Source: three-view drawing plus pictorial views. Frame: mm from the lowest corner of the part. A direction names the side the tool comes from. Give positions to 0.01 mm unless a question says otherwise; leave off trailing zeros. Write each loop counter-clockwise with the first axis right and the second up, starting at its lowest first coordinate (ties: lowest second). Pieces come first, ordered by that corner, then holes. Notation, with made-up numbers: (48.5, -31) - (76.5, -31) arc R13 ccw to (76.5, -10) - close; hole circle Ø9 at (85.5, 2). An arc over 180 degrees is marked (long way). One line per question, with ' | ' between items. Start each with the question number.
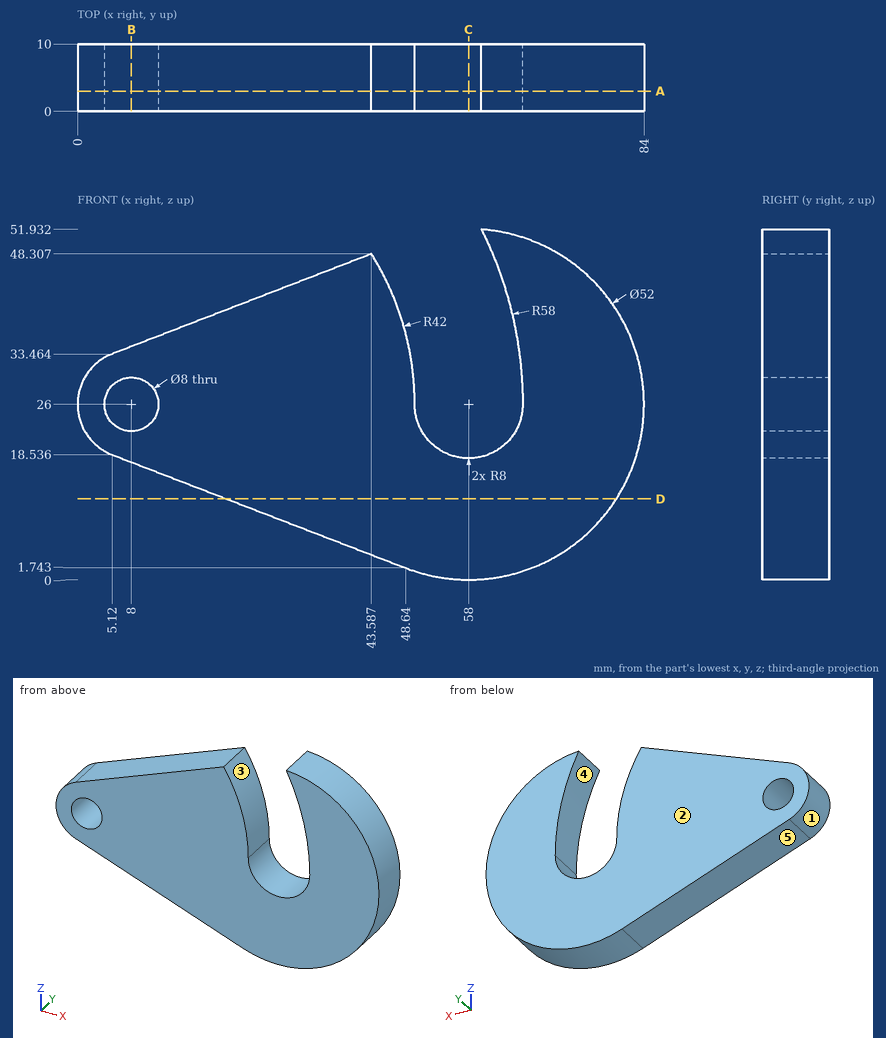
1) Section C-C, the plane x = 58. Output: boundary loops of the cut face in (y, z), plus the area to 3 significant figures.
2) First-contact query: pin 1 Ø4 at (y, z) = (2, 14.5) entering from +X; pin 2 Ø2 at (x, z) = (65.5, 27.5) entering from -Y; pin 3 Ø1.5 at (y, z) = (8.5, 32.5) entering from -X; pin 4 Ø4 at (y, z) = (6.5, 19) entering from +X (1 decimal). Flat tips, straight axial feed; report the tip coordinate or a pass-through.
3) Line query: L1, parallel to X at y = 8.5, z = 25.5 (1 decimal); L2, parallel to X at y = 3, z = 23 (1 decimal); L3, parallel to Z at x = 31.5, y = 7. Output: solid intervals per line, ascending.
4) Reachability of the marked faces 4 and 5 from +Z, -Z, +X, -X, +Y, -Y: full face, straight path, thin tool, end or side. Return the list, or none.
5) Pull-direction query (X, two-part tool) for the marked faces 1, 2 and 3; classes: +X half, -X half, draft (parallel to the pull), parting line (faces both ways), or undercut.
6) Section A-A, the plane y = 3. Output: boundary loops of the cut face in (x, z), plus the area to 3 significant figures.
7) Section D-D, the plane z = 12. Output: boundary loops of the cut face in (x, y).
8) Section B-B, the plane x = 8. Output: boundary loops of the cut face in (y, z) (1 decimal).
Answer key:
1) outline: (0, 0) - (10, 0) - (10, 18) - (0, 18) - close | area: 180 mm^2
2) pin 1: x = 82.2 | pin 2: y = 0 | pin 3: x = 2.44 | pin 4: x = 83.5
3) L1: 0 to 4, 12 to 50, 66 to 84 | L2: 0.6 to 5.4, 10.6 to 50.6, 65.4 to 83.8 | L3: 8.36 to 43.64
4) face 4: +Y, -Y | face 5: -Z, -X, +Y, -Y
5) face 1: -X half | face 2: draft | face 3: undercut
6) outline: (5.12, 18.54) - (48.64, 1.74) arc R26 ccw (long way) to (59.88, 51.93) arc R58 cw to (66, 26) arc R8 cw to (50, 26) arc R42 ccw to (43.59, 48.31) - (5.12, 33.46) arc R8 ccw to start; hole circle Ø8 at (8, 26) | area: 2,410 mm^2
7) outline: (22.06, 0) - (79.91, 0) - (79.91, 10) - (22.06, 10) - close
8) outline: (0, 17.4) - (10, 17.4) - (10, 22) - (0, 22) - close; (0, 30) - (10, 30) - (10, 34.6) - (0, 34.6) - close
